Design review of the part built by this model. Coordinates are the model's own, in mm. Face numbers are marked on the shaded views. A direction names the side the tool comes from. Give positions to 0.01 mm unless a question says otherwise; leave off trailing zeros. Write each loop counter-clockwise with the first axis right and the second up, starting at its lowest first coordinate (ties: lowest second). Pieces come first, ordered by that corner, then holes. Notation, with made-up numbers: (48.25, -31) -> (67.25, -31) arc R27 ccw to (67.25, -15) -> close; hole circle Ø2 at (62, -2). An arc over 180 degrees is marked (long way). Put each result on its own line as item: value. Start each with the question number.
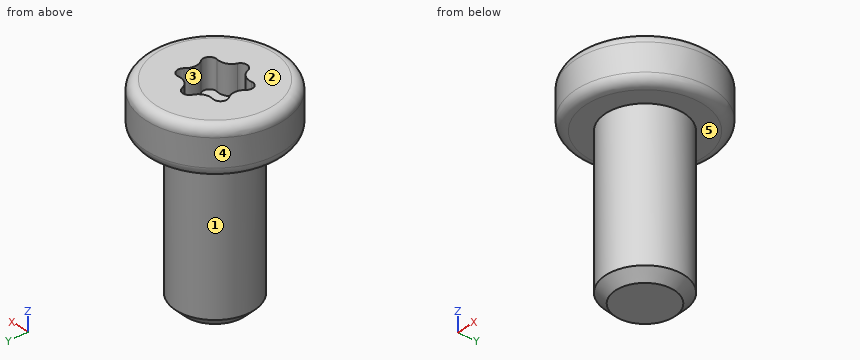
from build123d import *

# Parameters (mm, degrees)
F0_R     = 2
F1_DEPTH = 8
F2_R     = 3.5
F3_DEPTH = 2.4
F4_R     = 0.5
F5_SIZE  = 0.5
F7_DEPTH = 1.5


with BuildPart() as f1:
    # F0 (on Top) → F1 (new body)
    with BuildSketch(Plane.XY):
        Circle(F0_R)
    extrude(amount=F1_DEPTH)

    # F2 (on face) → F3 (join)
    with BuildSketch(Plane.XY.offset(8)):
        Circle(F2_R)
    extrude(amount=F3_DEPTH)

    # F4
    f4_edges = [f1.edges().sort_by_distance(p)[0] for p in [
        (-3.5, 0, 10.4),
        (-3.5, 0, 8),
    ]]
    fillet(f4_edges, radius=F4_R)

    # F5
    f5_edges = [f1.edges().sort_by_distance(p)[0] for p in [
        (-2, 0, 0),
    ]]
    chamfer(f5_edges, length=F5_SIZE)

    # F6 (on face) → F7 (cut)
    with BuildSketch(Plane.XY.offset(10.4)):
        with BuildLine():
            ThreePointArc((1.05752, 0.981425), (0.610199, 1.056896), (0.321179, 1.406552))
            ThreePointArc((0.321179, 1.406552), (0, 1.635), (-0.321179, 1.406552))
            ThreePointArc((-0.321179, 1.406552), (-0.610199, 1.056896), (-1.05752, 0.981425))
            ThreePointArc((-1.05752, 0.981425), (-1.415952, 0.8175), (-1.378699, 0.425126))
            ThreePointArc((-1.378699, 0.425126), (-1.220398, 0), (-1.378699, -0.425126))
            ThreePointArc((-1.378699, -0.425126), (-1.415952, -0.8175), (-1.05752, -0.981425))
            ThreePointArc((-1.05752, -0.981425), (-0.610199, -1.056896), (-0.321179, -1.406552))
            ThreePointArc((-0.321179, -1.406552), (0, -1.635), (0.321179, -1.406552))
            ThreePointArc((0.321179, -1.406552), (0.610199, -1.056896), (1.05752, -0.981425))
            ThreePointArc((1.05752, -0.981425), (1.415952, -0.8175), (1.378699, -0.425126))
            ThreePointArc((1.378699, -0.425126), (1.220398, 0), (1.378699, 0.425126))
            ThreePointArc((1.378699, 0.425126), (1.415952, 0.8175), (1.05752, 0.981425))
        make_face()
    extrude(amount=-F7_DEPTH, mode=Mode.SUBTRACT)


solid = f1.part
Q1. Take a section at C-C on z = 5. Give the boundary of the cut face in (x, y).
Q2. Mouldability with a two-part tool opening along X and no side actions: class the marked faces 1, 2 and 3 as +X half, -X half, draft (parallel to the pull), parting line (faces both ways), or undercut.
Q3. Take a section at B-B on x = 0. Give the boundary of the cut face in (y, z) (3 decimals).
Q4. Take a section at A-A on y = 0. Give the boundary of the cut face in (x, z).
Q5. To check wall thickness, follow probe 1 along Z at (x, y) = (-1.5, 1.5); probe 2 along Z at (x, y) = (0, -1); probe 3 along X at (y, z) = (-1.75, 2.5). State the ranges of each line that lie inside material, in increasing order. Write a range as from..to.
Q6. For pin 1 (1.5 mm diameter, centred on x = -1.5, z = 6.5, fed in from -Y), flat-tipped, find the tip position at first contact; note if it passes through.
Q7. Machinability: for the marked faces 4 and 5, which of the approach directions +Z, -Z, +X, -X, +Y, -Y give a long, thin tool a straight path to every point of the face, cutting with its end or side? Answer none if there is none.
Result:
1. outline: circle Ø4 at (0, 0)
2. face 1: parting line
2. face 2: draft
2. face 3: undercut
3. outline: (-3.5, 8.5) arc R0.5 ccw to (-3, 8) -> (-2, 8) -> (-2, 0.5) -> (-1.5, 0) -> (1.5, 0) -> (2, 0.5) -> (2, 8) -> (3, 8) arc R0.5 ccw to (3.5, 8.5) -> (3.5, 9.9) arc R0.5 ccw to (3, 10.4) -> (1.635, 10.4) -> (1.635, 8.9) -> (-1.635, 8.9) -> (-1.635, 10.4) -> (-3, 10.4) arc R0.5 ccw to (-3.5, 9.9) -> close
4. outline: (-3.5, 8.5) arc R0.5 ccw to (-3, 8) -> (-2, 8) -> (-2, 0.5) -> (-1.5, 0) -> (1.5, 0) -> (2, 0.5) -> (2, 8) -> (3, 8) arc R0.5 ccw to (3.5, 8.5) -> (3.5, 9.9) arc R0.5 ccw to (3, 10.4) -> (1.22, 10.4) -> (1.22, 8.9) -> (-1.22, 8.9) -> (-1.22, 10.4) -> (-3, 10.4) arc R0.5 ccw to (-3.5, 9.9) -> close
5. probe 1: z = 8..10.4
5. probe 2: z = 0..8.9
5. probe 3: x = -0.97..0.97
6. pin 1: stops at y = -1.85
7. face 4: +Z, -Z
7. face 5: -Z
